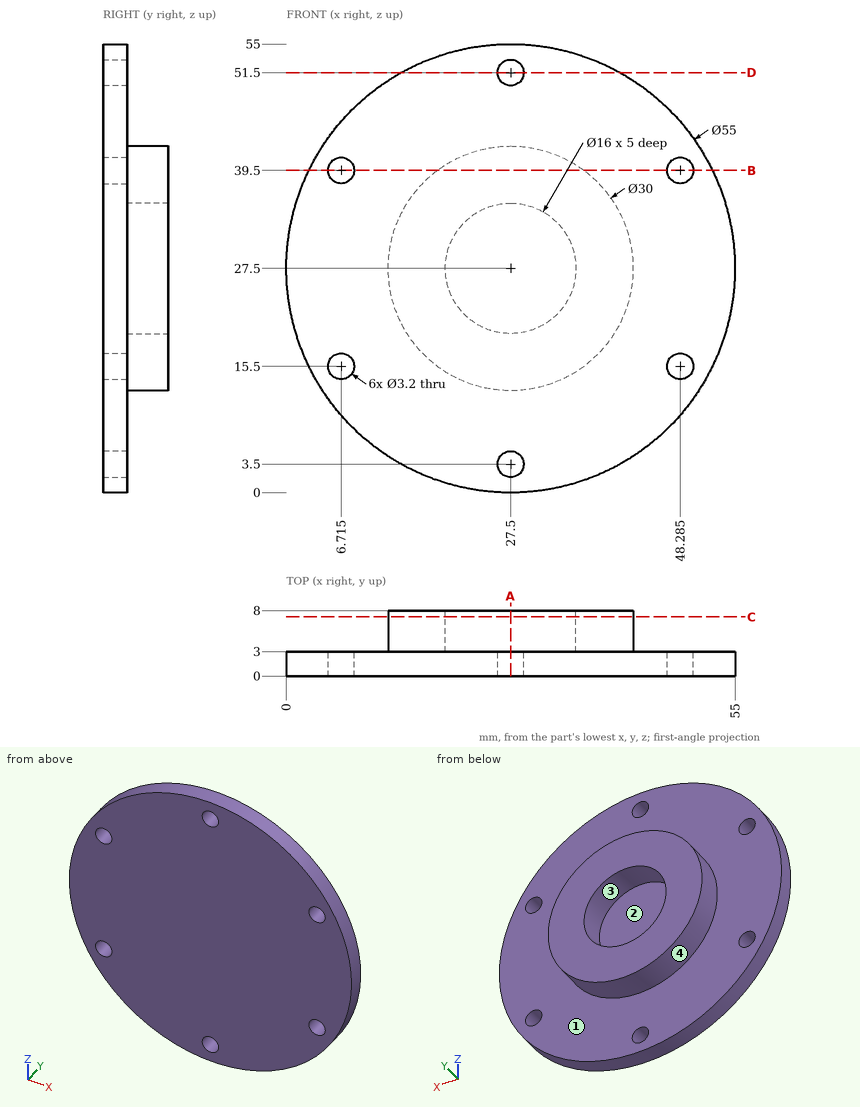
Design review of the part shown in the three views and the two pictorial views. Dimensions are in mm from the part's minimum x, y and z. Coordinates: 2 decimals unless noted, no trailing zeros. Write each loop counter-clockwise with the first axis right and the second up, starting at its lowest first coordinate (ties: lowest second). Pieces come first, ordered by that corner, then holes. Notation, with made-up numbers: (20.5, 60.25) -> (59.5, 60.25) arc R12 ccw to (59.5, 77.25) -> close; hole circle Ø1 at (48, 53.5). An arc over 180 degrees is marked (long way). Answer in a Markdown table with one row per item.
1. We need section A-A, the plane x = 27.5. State the section outline as (y, z) points.
Answers below:
| item | result |
|---|---|
| outline | (0, 0) -> (3, 0) -> (3, 1.9) -> (0, 1.9) -> close; (0, 5.1) -> (3, 5.1) -> (3, 12.5) -> (8, 12.5) -> (8, 19.5) -> (3, 19.5) -> (3, 35.5) -> (8, 35.5) -> (8, 42.5) -> (3, 42.5) -> (3, 49.9) -> (0, 49.9) -> close; (0, 53.1) -> (3, 53.1) -> (3, 55) -> (0, 55) -> close |
2. We need section C-C, the plane y = 7.25. State the section outline as (x, z) points, and give its area (3 significant figures).
Answers below:
| item | result |
|---|---|
| outline | circle Ø30 at (27.5, 27.5); hole circle Ø16 at (27.5, 27.5) |
| area | 506 mm^2 |
3. Clearance check with flat-ended pins moving along their axes: pin 1 Ø1 at (x, z) = (16, 42.5) entering from +Y; pin 2 Ø4 at (x, y) = (16.5, 2) entering from +Z (1 decimal); pin 3 Ø2.5 at (x, z) = (27.5, 51.5) entering from -Y; pin 4 Ø1.5 at (x, y) = (40, 6) entering from -Z (1 decimal). State where each tip first meets the part, or that it passes through.
Answers below:
| item | result |
|---|---|
| pin 1 | stops at y = 3 |
| pin 2 | stops at z = 53.5 |
| pin 3 | passes through |
| pin 4 | stops at z = 18.2 |
4. Draft analysis for pull direction Z (two halves, no side actions). For the marked faces 1, 2, 3 and 4, state which applies: +Z half, -Z half, draft (parallel to the pull), parting line (faces both ways), or undercut.
Answers below:
| item | result |
|---|---|
| face 1 | draft |
| face 2 | undercut |
| face 3 | undercut |
| face 4 | parting line |
5. We need section B-B, the plane z = 39.5. State the section outline as (x, y) points (1 decimal).
Answers below:
| item | result |
|---|---|
| outline | (2.8, 0) -> (5.1, 0) -> (5.1, 3) -> (2.8, 3) -> close; (8.3, 0) -> (46.7, 0) -> (46.7, 3) -> (36.5, 3) -> (36.5, 8) -> (18.5, 8) -> (18.5, 3) -> (8.3, 3) -> close; (49.9, 0) -> (52.2, 0) -> (52.2, 3) -> (49.9, 3) -> close |
6. We need section D-D, the plane z = 51.5. State the section outline as (x, y) points (1 decimal).
Answers below:
| item | result |
|---|---|
| outline | (14.1, 0) -> (25.9, 0) -> (25.9, 3) -> (14.1, 3) -> close; (29.1, 0) -> (40.9, 0) -> (40.9, 3) -> (29.1, 3) -> close |
7. Wall thickness on probe 1 along X at (y, z) = (2.1, 15.5) (1 decimal); probe 2 along Z at (x, y) = (27, 1.75) (1 decimal); probe 3 along Y at (x, z) = (43.5, 18): over which ranges is each line inside the solid? List them lowest first. Write a range as [from, to].
Answers below:
| item | result |
|---|---|
| probe 1 | x = [2.8, 5.1], [8.3, 46.7], [49.9, 52.2] |
| probe 2 | z = [0, 2], [5, 50], [53, 55] |
| probe 3 | y = [0, 3] |
